from build123d import *

# Parameters (mm, degrees)
SKETCH_1_W          = 43
SKETCH_1_H          = 30
SKETCH_1_R          = 4.25
EXTRUDE_1_DEPTH     = 3
SKETCH_2_W          = 6
SKETCH_2_H          = 14
CUT_EXTRUDE_1_DEPTH = 3
CUT_EXTRUDE_2_REACH = 5
SKETCH_3_R          = 1.25


with BuildPart() as part:
    # 草图1 → 凸台-拉伸1 (new body)
    with BuildSketch(Plane(origin=(0, 0, 0), x_dir=(1, 0, 0), z_dir=(0, 1, 0))):
        Rectangle(SKETCH_1_W, SKETCH_1_H)
        Circle(SKETCH_1_R, mode=Mode.SUBTRACT)
    extrude(amount=EXTRUDE_1_DEPTH)

    # 草图2 → 切除-拉伸1 (cut)
    with BuildSketch(Plane(origin=(0, 3, 0), x_dir=(1, 0, 0), z_dir=(0, 1, 0))):
        with Locations((21.5, 0)):
            Rectangle(SKETCH_2_W, SKETCH_2_H)
        with Locations((-21.5, 0)):
            Rectangle(SKETCH_2_W, SKETCH_2_H)
    extrude(amount=-CUT_EXTRUDE_1_DEPTH, mode=Mode.SUBTRACT)

    # 草图3 → 切除-拉伸2 (cut, up to next)
    with BuildSketch(Plane.XZ, mode=Mode.PRIVATE) as cut_extrude_2_sk1:
        with Locations((-18.5, 5.75)):
            Circle(SKETCH_3_R)
    cut_extrude_2_tool1 = extrude(cut_extrude_2_sk1.sketch, amount=-CUT_EXTRUDE_2_REACH, mode=Mode.PRIVATE) & part.part
    add(cut_extrude_2_tool1.solids().sort_by_distance((-18.5, 0, 5.75))[0], mode=Mode.SUBTRACT)
    # 草图3 → 切除-拉伸2 (cut, up to next)
    with BuildSketch(Plane.XZ, mode=Mode.PRIVATE) as cut_extrude_2_sk2:
        with Locations((-18.5, -5.75)):
            Circle(SKETCH_3_R)
    cut_extrude_2_tool2 = extrude(cut_extrude_2_sk2.sketch, amount=-CUT_EXTRUDE_2_REACH, mode=Mode.PRIVATE) & part.part
    add(cut_extrude_2_tool2.solids().sort_by_distance((-18.5, 0, -5.75))[0], mode=Mode.SUBTRACT)
    # 草图3 → 切除-拉伸2 (cut, up to next)
    with BuildSketch(Plane.XZ, mode=Mode.PRIVATE) as cut_extrude_2_sk3:
        with Locations((18.5, -5.75)):
            Circle(SKETCH_3_R)
    cut_extrude_2_tool3 = extrude(cut_extrude_2_sk3.sketch, amount=-CUT_EXTRUDE_2_REACH, mode=Mode.PRIVATE) & part.part
    add(cut_extrude_2_tool3.solids().sort_by_distance((18.5, 0, -5.75))[0], mode=Mode.SUBTRACT)
    # 草图3 → 切除-拉伸2 (cut, up to next)
    with BuildSketch(Plane.XZ, mode=Mode.PRIVATE) as cut_extrude_2_sk4:
        with Locations((18.5, 5.75)):
            Circle(SKETCH_3_R)
    cut_extrude_2_tool4 = extrude(cut_extrude_2_sk4.sketch, amount=-CUT_EXTRUDE_2_REACH, mode=Mode.PRIVATE) & part.part
    add(cut_extrude_2_tool4.solids().sort_by_distance((18.5, 0, 5.75))[0], mode=Mode.SUBTRACT)


solid = part.part
The model under review builds one solid part; all positions refer to its coordinate system, in mm. A direction names the side the tool comes from. Coordinates: 2 decimals unless noted, no trailing zeros. Order: outer loops, then holes, each group sorted by start corner. A loop starts at its lowest first (then second) coordinate and runs counter-clockwise, first axis right, second up. Notation, with made-up numbers: (53.25, -28.5) -> (65.25, -28.5) arc R20 cw to (65.25, 9.5) -> close; hole circle Ø4 at (-28.5, 11.5). An arc over 180 degrees is marked (long way). Answer in a Markdown table with one row per item.
(1) The part is to be moulded in two halves that separate along X. For faces 1 (the flat face through (21.5, 1, -11)), 2 (the cylindrical face through (-17.25, 1.48, 5.72)), 3 (the cylindrical face through (2.285, 1.479, -3.584)), 4 (the flat face through (20, 2, 7)), say which applies: +X half, -X half, draft (parallel to the pull), parting line (faces both ways), or undercut.
Answers:
| item | result |
|---|---|
| face 1 | +X half |
| face 2 | -X half |
| face 3 | undercut |
| face 4 | draft |
(2) Consider section D-D (z = 5.75). Write out the cut boundary in (x, y), plus the area to 4 significant figures.
Answers:
| item | result |
|---|---|
| outline | (-17.25, 0) -> (17.25, 0) -> (17.25, 3) -> (-17.25, 3) -> close |
| area | 103.5 mm² |
(3) Machinability: for faces 5 (the flat face through (-20, 2, 7)), 6 (the flat face through (-21.5, 1, -11)), 7 (the flat face through (20, 2, -7)), which of the approach directions +Z, -Z, +X, -X, +Y, -Y give a long, thin tool a straight path to every point of the face, cutting with its end or side? Answer none if there is none.
Answers:
| item | result |
|---|---|
| face 5 | -X, +Y, -Y |
| face 6 | +Z, -Z, -X, +Y, -Y |
| face 7 | +X, +Y, -Y |
(4) Consider section C-C (x = 3). Write out the cut boundary in (y, z), plus the area to 3 significant figures.
Answers:
| item | result |
|---|---|
| outline | (0, -15) -> (3, -15) -> (3, -3.01) -> (0, -3.01) -> close; (0, 3.01) -> (3, 3.01) -> (3, 15) -> (0, 15) -> close |
| area | 71.9 mm² |
(5) Wall thickness on line 1 along X through (y, z) = (1.4, 0); line 2 along Z through (x, y) = (18, 2.45); line 3 along X through (y, z) = (2.25, 5.75): over which ranges is each line inside the solid? List them lowest first.
Answers:
| item | result |
|---|---|
| line 1 | -18.5 to -4.25, 4.25 to 18.5 |
| line 2 | -15 to -6.9, -4.6 to 4.6, 6.9 to 15 |
| line 3 | -17.25 to 17.25 |
(6) Insertion check: pin 1 (1.5 mm diameter, centred on y = 1, z = 2, fed in from +X); pin 2 (1.5 mm diameter, centred on y = 1, z = -2, fed in from -X). Each pin has a flat end and moves straight along its axis. Give the tip position at first contact, or say it passes through.
Answers:
| item | result |
|---|---|
| pin 1 | x = 18.5 |
| pin 2 | x = -18.5 |
(7) Consider section B-B (y = 1.95). Write out the cut boundary in (x, z).
Answers:
| item | result |
|---|---|
| outline | (-21.5, -15) -> (21.5, -15) -> (21.5, -7) -> (18.5, -7) arc R1.25 cw to (18.5, -4.5) -> (18.5, 4.5) arc R1.25 cw to (18.5, 7) -> (21.5, 7) -> (21.5, 15) -> (-21.5, 15) -> (-21.5, 7) -> (-18.5, 7) arc R1.25 cw to (-18.5, 4.5) -> (-18.5, -4.5) arc R1.25 cw to (-18.5, -7) -> (-21.5, -7) -> close; hole circle Ø8.5 at (0, 0) |
(8) Consider section A-A (z = 0). Write out the cut boundary in (x, y), plus the area to 3 significant figures.
Answers:
| item | result |
|---|---|
| outline | (-18.5, 0) -> (-4.25, 0) -> (-4.25, 3) -> (-18.5, 3) -> close; (4.25, 0) -> (18.5, 0) -> (18.5, 3) -> (4.25, 3) -> close |
| area | 85.5 mm² |
